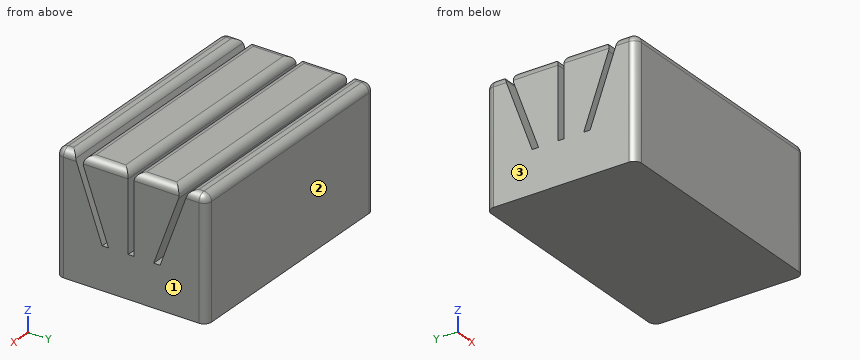
```python
from build123d import *

# Parameters (mm, degrees)
F0_W     = 160
F0_H     = 100
F1_DEPTH = 80
F2_W     = 4
F2_H     = 52
F3_DEPTH = 160
F4_R     = 5


with BuildPart() as f1:
    # F0 (on Top) → F1 (new body)
    with BuildSketch(Plane.XY):
        with Locations((80, 50)):
            Rectangle(F0_W, F0_H)
    extrude(amount=F1_DEPTH)

    # F2 (on face) → F3 (cut, through all)
    with BuildSketch(Plane(origin=(0, 0, 0), x_dir=(0, -1, 0), z_dir=(-1, 0, 0))):
        Polygon((-65.0198098907, 28), (-83.9462620725, 80), (-88.2029731624, 80), (-69.2765209806, 28), align=None)
        with Locations((-50, 54)):
            Rectangle(F2_W, F2_H)
        Polygon((-30.7234790194, 28), (-11.7970268376, 80), (-16.0537379275, 80), (-34.9801901093, 28), align=None)
    extrude(amount=-F3_DEPTH, mode=Mode.SUBTRACT)

    # F4
    f4_edges = [f1.edges().sort_by_distance(p)[0] for p in [
        (80, 0, 80),
        (80, 100, 80),
        (160, 94.101487, 80),
        (160, 67.973131, 80),
        (160, 32.026869, 80),
        (160, 5.898513, 80),
        (0, 5.898513, 80),
        (0, 32.026869, 80),
        (0, 67.973131, 80),
        (0, 94.101487, 80),
        (160, 100, 40),
        (0, 100, 40),
        (160, 0, 40),
        (0, 0, 40),
        (80, 48, 80),
        (80, 52, 80),
        (80, 83.946262, 80),
        (80, 88.202973, 80),
        (80, 16.053738, 80),
        (80, 11.797027, 80),
    ]]
    fillet(f4_edges, radius=F4_R)


solid = f1.part
```
Check sheet for the modelled part. Datum: model origin and axes. Units: mm. Face numbers are marked on the shaded views. Round coordinates to 2 decimals unless told otherwise and drop trailing zeros. Write each loop counter-clockwise with the first axis right and the second up, starting at its lowest first coordinate (ties: lowest second). Pieces come first, ordered by that corner, then holes. Notation, with made-up numbers: (-26, 57.5) -> (18, 57.5) arc R36 ccw to (18, 96.5) -> close; hole circle Ø9 at (22, 2). An arc over 180 degrees is marked (long way). Put each result on its own line as item: value.
(1) Mould release check, pull along X, two halves, no side actions. Record for the marked faces 1, 2 and 3: released by +X, released by -X, zero draft, split by the parting line, or undercut.
Values found:
face 1: released by +X
face 2: zero draft
face 3: released by -X
(2) Sectioned sample at C-C (x = 74.5). Enter the section's corners in (y, z), plus the area to 3 significant figures.
Values found:
outline: (0, 0) -> (100, 0) -> (100, 75) arc R5 ccw to (95, 80) -> (91.7, 80) arc R5 ccw to (87.01, 76.71) -> (69.28, 28) -> (65.02, 28) -> (81.5, 73.29) arc R5 ccw to (76.81, 80) -> (57, 80) arc R5 ccw to (52, 75) -> (52, 28) -> (48, 28) -> (48, 75) arc R5 ccw to (43, 80) -> (23.19, 80) arc R5 ccw to (18.5, 73.29) -> (34.98, 28) -> (30.72, 28) -> (12.99, 76.71) arc R5 ccw to (8.3, 80) -> (5, 80) arc R5 ccw to (0, 75) -> close
area: 7,300 mm^2
(3) Sectioned sample at A-A (z = 47). Enter the section's corners in (x, y), plus the area to 3 significant figures.
Values found:
outline: (0, 5) arc R5 ccw to (5, 0) -> (155, 0) arc R5 ccw to (160, 5) -> (160, 23.81) -> (0, 23.81) -> close; (0, 28.06) -> (160, 28.06) -> (160, 48) -> (0, 48) -> close; (0, 52) -> (160, 52) -> (160, 71.94) -> (0, 71.94) -> close; (0, 76.19) -> (160, 76.19) -> (160, 95) arc R5 ccw to (155, 100) -> (5, 100) arc R5 ccw to (0, 95) -> close
area: 14,000 mm^2
(4) Material ranges on line 1 (Y direction, x = 72, z = 44); line 2 (Y direction, x = 92, z = 54); line 3 (Z direction, x = 85, y = 43.5), recorded low to high.
Values found:
line 1: y = 0 to 24.9, 29.16 to 48, 52 to 70.84, 75.1 to 100
line 2: y = 0 to 21.26, 25.52 to 48, 52 to 74.48, 78.74 to 100
line 3: z = 0 to 79.97
(5) Sectioned sample at B-B (y = 28). Enter the section's corners in (x, z).
Values found:
outline: (0, 0) -> (160, 0) -> (160, 35.48) -> (0, 35.48) -> close; (0, 47.18) -> (160, 47.18) -> (160, 75) arc R5 ccw to (155, 80) -> (5, 80) arc R5 ccw to (0, 75) -> close
(6) Sectioned sample at D-D (y = 16). Enter the section's corners in (x, z).
Values found:
outline: (0, 0) -> (160, 0) -> (160, 68.45) -> (0, 68.45) -> close
